Part print with two shaded views. Sizes in mm from the minimum x, y, z corner. A direction names the side the tool comes from. Round coordinates to 2 decimals unless told otherwise and drop trailing zeros. Write each loop counter-clockwise with the first axis right and the second up, starting at its lowest first coordinate (ties: lowest second). Pieces come first, ordered by that corner, then holes. Notation, with made-up numbers: (13, 0) - (43, 0) arc R20 ccw to (43, 25) - close; hole circle Ø2 at (39, -37.75). An arc over 180 degrees is marked (long way). Answer as a JSON object with one key per item and string values. Group by question number.
Item 1: Probe line 1 (X direction, y = 3.75, z = 4.75); line 2 (Z direction, x = 1, y = 5.75). List the from-to ranges inside material, lowest first. Write a range as from..to.
Item 2: Slice it at A-A, the plane y = 4.75. List the corners of the cut face in (x, z) (1 decimal).
Item 3: Flat gauge pins, fed straight in: pin 1 (1.5 mm diameter, centred on y = 5.5, z = 19.5, fed in from +X) (1 decimal); pin 2 (1.4 mm diameter, centred on x = 4.5, z = 2, fed in from -Y); pin 3 (3 mm diameter, centred on x = 2.5, y = 5.5, fed in from +Z); pin 4 (1 mm diameter, centred on x = 6, y = 4, fed in from +Z). Where does each tip first touch, or does it go through?
Item 4: Slice it at C-C, the plane z = 21.75. List the corners of the cut face in (x, y) (1 decimal).
Item 5: Which spindle directions (+Z, -Z, +X, -X, +Y, -Y) get a long thin tool onto all of the face, cutting with end or side? Do the marked faces 1, 2, 3, 4 and 5. Say none if no direction does.
Item 6: Slice it at B-B, the plane x = 3.81. List the corners of the cut face in (y, z) (1 decimal).
Item 7: Slice it at D-D, the plane x = 6. List the corners of the cut face in (y, z).
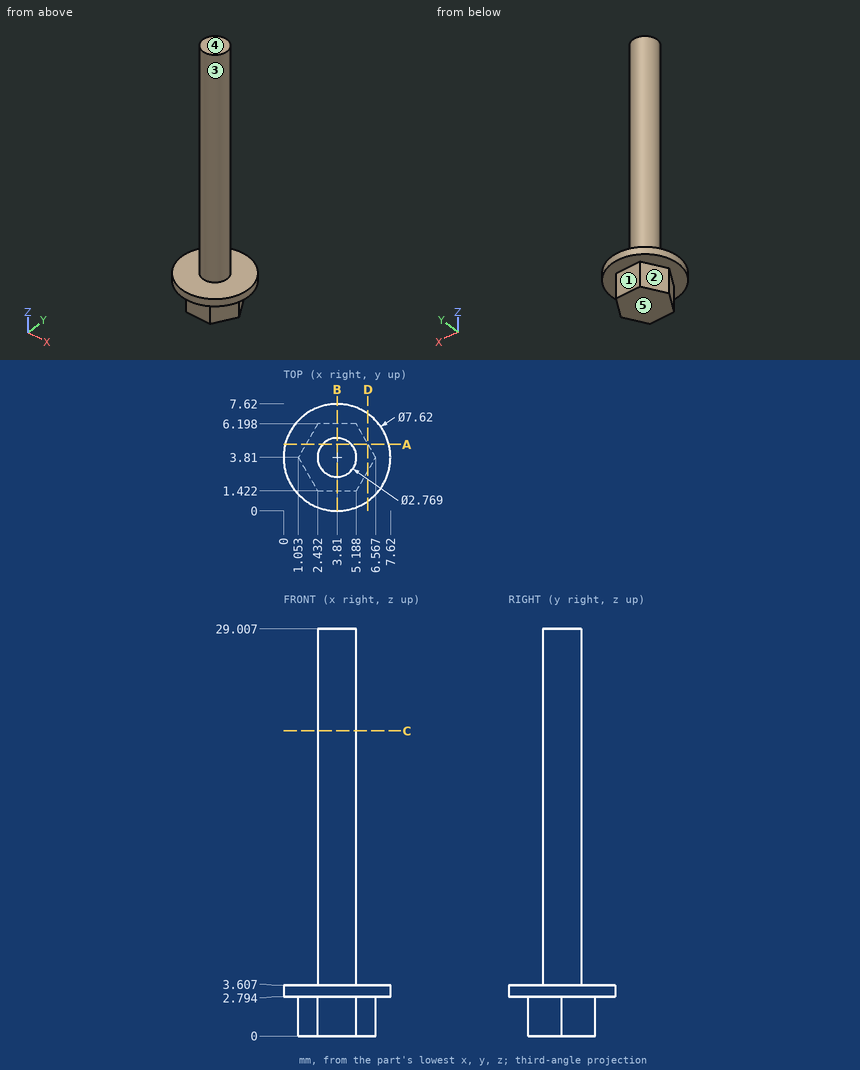
Geometry says:
{
 "1": {"line 1": "x = 2.43..5.19", "line 2": "z = 2.79..3.61"},
 "2": {"outline": "(0.1, 2.8) - (1.6, 2.8) - (1.6, 0) - (6, 0) - (6, 2.8) - (7.5, 2.8) - (7.5, 3.6) - (4.8, 3.6) - (4.8, 29) - (2.8, 29) - (2.8, 3.6) - (0.1, 3.6) - close"},
 "3": {"pin 1": "stops at x = 4.8", "pin 2": "stops at y = 1.42", "pin 3": "stops at z = 29.01", "pin 4": "stops at z = 3.61"},
 "4": {"outline": "circle Ø2.8 at (3.8, 3.8)"},
 "5": {"face 1": "-Z, +X, -X, +Y", "face 2": "-Z, -X, +Y", "face 3": "+Z", "face 4": "+Z, +X, -X, +Y, -Y", "face 5": "-Z, +X, -X, +Y, -Y"},
 "6": {"outline": "(0, 2.8) - (1.4, 2.8) - (1.4, 0) - (6.2, 0) - (6.2, 2.8) - (7.6, 2.8) - (7.6, 3.6) - (5.2, 3.6) - (5.2, 29) - (2.4, 29) - (2.4, 3.6) - (0, 3.6) - close"},
 "7": {"outline": "(0.69, 2.79) - (2.83, 2.79) - (2.83, 0) - (4.79, 0) - (4.79, 2.79) - (6.93, 2.79) - (6.93, 3.61) - (0.69, 3.61) - close"}
}
